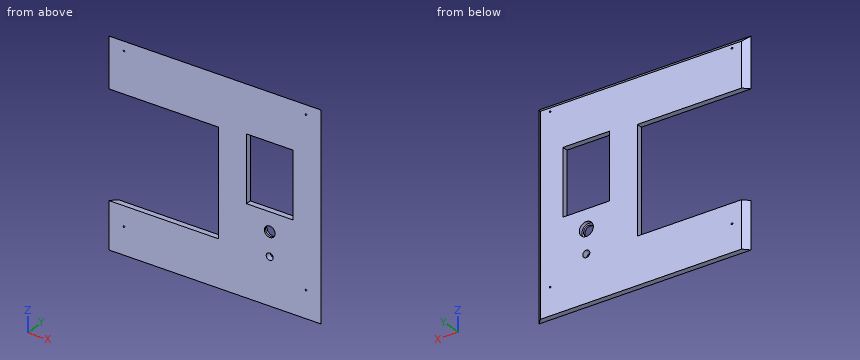
```python
from build123d import *

# Parameters (mm, degrees)
F0_W     = 454
F0_H     = 429
F1_DEPTH = 12
F2_SIZE  = 11.99999
F3_W     = 235
F3_H     = 224
F3_W_2   = 100
F3_H_2   = 140
F3_R     = 11.5
F3_R_2   = 7.5
F4_DEPTH = 25
F6_D     = 3.5
F7_R     = 15
F7_R_2   = 11.5
F8_DEPTH = 8


# Not quite as in the source:
# - a fillet or chamfer is up to 0.001 mm smaller than in the source, because OpenCascade refuses the exact size


with BuildPart() as f1:
    # F0 (on Front) → F1 (new body)
    with BuildSketch(Plane.XZ):
        Rectangle(F0_W, F0_H)
    extrude(amount=F1_DEPTH)

    # F2 (size 12 in the source; OpenCascade refuses exactly that, so slightly less here)
    f2_edges = [f1.edges().sort_by_distance(p)[0] for p in [
        (227, 0, 0),
        (-227, 0, 0),
        (0, 0, 214.5),
    ]]
    chamfer(f2_edges, length=F2_SIZE)

    # F3 (on face) → F4 (cut)
    with BuildSketch(Plane.XZ.offset(12)):
        with Locations((-109.5, -3.5)):
            Rectangle(F3_W, F3_H)
        with Locations((117, 44.5)):
            Rectangle(F3_W_2, F3_H_2)
        with Locations((117, -65.5)):
            Circle(F3_R)
        with Locations((117, -115.5)):
            Circle(F3_R_2)
    extrude(amount=-F4_DEPTH, mode=Mode.SUBTRACT)

    # F6 (through all)
    with Locations(Plane.XZ.offset(12)):
        with Locations((-194.5, 195), (194.5, 195), (194.5, -157), (-194.5, -157)):
            Hole(F6_D / 2)

    # F7 (on face) → F8 (cut)
    with BuildSketch(Plane(origin=(0, 0, 0), x_dir=(-1, 0, 0), z_dir=(0, 1, 0))):
        with Locations((-117, -65.5)):
            Circle(F7_R)
        with Locations((-117, -65.5)):
            Circle(F7_R_2, mode=Mode.SUBTRACT)
    extrude(amount=-F8_DEPTH, mode=Mode.SUBTRACT)


solid = f1.part
```
Build history of the part. All positions in model axes, mm. Coordinates: 2 decimals unless noted, no trailing zeros. Order: outer loops, then holes, each group sorted by start corner. A loop starts at its lowest first (then second) coordinate and runs counter-clockwise, first axis right, second up. Notation, with made-up numbers: M 74.5,-30.75 L 132.5,-30.75 A25 cw 132.5,-4.75 Z; hole C -32.5,46.5 d10. An arc over 180 degrees is marked long. One line per question, with ' | ' between items. Start each with the question number.
1. Cut at C-C (y = -3). Write the cut outline in (x, z).
2. Wall check: line 1 along Z through (x, y) = (117, -9.35); line 2 along Z through (x, y) = (117, -11.2); line 3 along Z through (x, y) = (96, -3). Give the ranges that are in metal, low to high. Write a range as [from, to].
3. Flat gauge pins, fed straight in: P1, Ø5.5, axis at x = 194.5, z = -157, coming from the +Y side; P2, Ø3, axis at y = -4.5, z = 33, coming from the -X side; P3, Ø3.5, axis at x = -59.5, y = -4.5, coming from the +Z side; P4, Ø5, axis at y = -10.5, z = 126.5, coming from the +X side. Where does each tip first touch, or does it go through?
4. Cut at A-A (x = 117). Count the separate pieces of the cut face and the enclosed holes in it, plus the area to 3 significant figures.
The answers:
1) outline: M -218,-214.5 L 218,-214.5 L 218,205.5 L -218,205.5 L -218,108.5 L 8,108.5 L 8,-115.5 L -218,-115.5 Z; hole C -194.5,-157 d3.5; hole C -194.5,195 d3.5; hole M 67,-25.5 L 167,-25.5 L 167,114.5 L 67,114.5 Z; hole C 117,-65.5 d30; hole C 117,-115.5 d15; hole C 194.5,-157 d3.5; hole C 194.5,195 d3.5
2) line 1: z = [-214.5, -123], [-108, -77], [-54, -25.5], [114.5, 211.85] | line 2: z = [-214.5, -123], [-108, -77], [-54, -25.5], [114.5, 213.7] | line 3: z = [-214.5, -25.5], [114.5, 205.5]
3) P1: stops at y = 0 | P2: stops at x = 8 | P3: stops at z = 208.75 | P4: stops at x = 227
4) separate pieces: 4 | enclosed holes: 0 | area: 2,880 mm2
